Part model, mm, in its own coordinate system. Face numbers are marked on the shaded views. Round coordinates to 2 decimals unless told otherwise and drop trailing zeros. Loops run counter-clockwise (first coordinate to the right, second up) from the corner with the lowest first, then second, coordinate; pieces in that order, holes last. Notation, with made-up numbers: (-26.5, 2.25) -> (0.5, 2.25) arc R16 ccw to (0.5, 31.25) -> close; hole circle Ø7 at (82.5, -20.5). An arc over 180 degrees is marked (long way). Use a Markdown table: item, result. Add a question column.
Item 1: Cut at B-B, the plane y = -3.75. List the corners of the cut face in (x, z), plus the area to 3 significant figures.
Item 2: Flat gauge pins, fed straight in: pin 1 (1.9 mm diameter, centred on x = 0, z = 0, fed in from -Y); pin 2 (2 mm diameter, centred on y = -3.5, z = -3.5, fed in from -X); pin 3 (4 mm diameter, centred on x = 0, z = 0, fed in from -Y); pin 4 (1 mm diameter, centred on x = 4.5, y = -5, fed in from -Z). Where does each tip first touch, or does it go through?
Item 3: Cut at A-A, the plane z = -8. List the corners of the cut face in (x, y), plus the area to 3 significant figures.
Item 4: Cut at D-D, the plane z = 0. List the corners of the cut face in (x, y).
Item 5: Two-plate mould, pull along X, no slides. Class the marked faces 1, 2, 3 and 4: pulls with the +X half, pulls with the -X half, needs draft (parallel to the pull), parting line crosses it, or undercut.
Item 6: Cut at C-C, the plane x = -1.25. List the corners of the cut face in (y, z), plus the area to 3 significant figures.
Item 7: Probe line 1 (X direction, y = -4, z = -4.75); line 2 (Z direction, x = -6.5, y = -5.5); line 3 (Z direction, x = 7, y = -4.5). List the from-to ranges inside material, lowest first. Write a range as [from, to].
```python
from build123d import *

# Parameters (mm, degrees)
F0_R          = 12.7
F0_R_2        = 2
F0_R_3        = 1.5875
F1_DEPTH      = 6
F2_R          = 2
F3_DEPTH      = 12.701
F3_DEPTH_BACK = 12.701


with BuildPart() as f1:
    # F0 (on Front) → F1 (new body)
    with BuildSketch(Plane.XZ):
        Circle(F0_R)
        with Locations((-6.3639610307, -6.3639610307)):
            Circle(F0_R_2, mode=Mode.SUBTRACT)
        Circle(F0_R_3, mode=Mode.SUBTRACT)
        with Locations((6.3639610307, -6.3639610307)):
            Circle(F0_R_2, mode=Mode.SUBTRACT)
        with Locations((-6.3639610307, 6.3639610307)):
            Circle(F0_R_2, mode=Mode.SUBTRACT)
        with Locations((6.3639610307, 6.3639610307)):
            Circle(F0_R_2, mode=Mode.SUBTRACT)
    extrude(amount=F1_DEPTH)

    # F2 (on Top) → F3 (cut, two sides)
    with BuildSketch(Plane.XY) as f3_sk:
        with Locations((0, -3)):
            Circle(F2_R)
    extrude(amount=-F3_DEPTH, mode=Mode.SUBTRACT)
    extrude(f3_sk.sketch, amount=F3_DEPTH_BACK, mode=Mode.SUBTRACT)


solid = f1.part
```
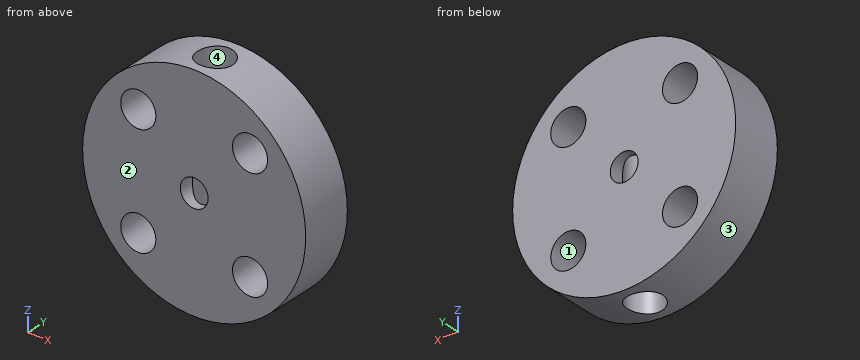
A:
| question | item | result |
|---|---|---|
| 1 | outline | (-1.85, -12.56) -> (-1.85, 12.56) arc R12.7 ccw to start; (1.85, -12.56) arc R12.7 ccw to (1.85, 12.56) -> close; hole circle Ø4 at (-6.36, -6.36); hole circle Ø4 at (-6.36, 6.36); hole circle Ø4 at (6.36, -6.36); hole circle Ø4 at (6.36, 6.36) |
| 1 | area | 363 mm^2 |
| 2 | pin 1 | passes through |
| 2 | pin 2 | stops at x = -12.45 |
| 2 | pin 3 | stops at y = -6 |
| 2 | pin 4 | stops at z = -12.05 |
| 3 | outline | (-9.86, -6) -> (-7.51, -6) -> (-7.51, 0) -> (-9.86, 0) -> close; (-5.21, -6) -> (5.21, -6) -> (5.21, 0) -> (-5.21, 0) -> close; (7.51, -6) -> (9.86, -6) -> (9.86, 0) -> (7.51, 0) -> close; hole circle Ø4 at (0, -3) |
| 3 | area | 78.2 mm^2 |
| 4 | outline | (-12.7, -6) -> (-1.59, -6) -> (-1.59, -4.22) arc R2 cw to (-1.59, -1.78) -> (-1.59, 0) -> (-12.7, 0) -> close; (1.59, -6) -> (12.7, -6) -> (12.7, 0) -> (1.59, 0) -> (1.59, -1.78) arc R2 cw to (1.59, -4.22) -> close |
| 5 | face 1 | undercut |
| 5 | face 2 | needs draft |
| 5 | face 3 | parting line crosses it |
| 5 | face 4 | undercut |
| 6 | outline | (-6, -12.64) -> (-4.56, -12.64) -> (-4.56, -0.98) -> (-6, -0.98) -> close; (-6, 0.98) -> (-4.56, 0.98) -> (-4.56, 12.64) -> (-6, 12.64) -> close; (-1.44, -12.64) -> (0, -12.64) -> (0, -0.98) -> (-1.44, -0.98) -> close; (-1.44, 0.98) -> (0, 0.98) -> (0, 12.64) -> (-1.44, 12.64) -> close |
| 6 | area | 67.1 mm^2 |
| 7 | line 1 | x = [-11.78, -7.55], [-5.18, -1.73], [1.73, 5.18], [7.55, 11.78] |
| 7 | line 2 | z = [-10.91, -8.36], [-4.37, 4.37], [8.36, 10.91] |
| 7 | line 3 | z = [-10.6, -8.26], [-4.47, 4.47], [8.26, 10.6] |
